```python
from build123d import *

# Parameters (mm, degrees)
F0_R     = 95.25
F0_R_2   = 31.75
F1_DEPTH = 50.8


with BuildPart() as f1:
    # F0 (on Front) → F1 (new body)
    with BuildSketch(Plane.XZ):
        Circle(F0_R)
        with BuildLine():
            ThreePointArc((46.990183, 59.986354), (65.491159, 38.953153), (75.141667, 12.655826))
            ThreePointArc((75.141667, 12.655826), (84.797941, 9.346947), (88.9, 0))
            ThreePointArc((88.9, 0), (84.797941, -9.346947), (75.141667, -12.655826))
            ThreePointArc((75.141667, -12.655826), (65.407135, -39.094076), (46.731427, -60.188153))
            ThreePointArc((46.731427, -60.188153), (48.087021, -63.052889), (48.552253, -66.187838))
            ThreePointArc((48.552253, -66.187838), (40.152635, -76.713719), (28.025311, -70.85917))
            ThreePointArc((28.025311, -70.85917), (0.009492, -76.199999), (-28.007657, -70.86615))
            ThreePointArc((-28.007657, -70.86615), (-43.08737, -75.575185), (-46.716431, -60.199793))
            ThreePointArc((-46.716431, -60.199793), (-65.887351, -38.279198), (-75.435354, -10.767885))
            ThreePointArc((-75.435354, -10.767885), (-86.995, 0), (-75.435354, 10.767885))
            ThreePointArc((-75.435354, 10.767885), (-66.114858, 37.884899), (-47.432359, 59.637332))
            ThreePointArc((-47.432359, 59.637332), (-43.987261, 75.054986), (-28.852362, 70.526458))
            ThreePointArc((-28.852362, 70.526458), (-0.281663, 76.199479), (28.330193, 70.737827))
            ThreePointArc((28.330193, 70.737827), (40.459969, 76.545328), (48.836928, 66.024629))
            ThreePointArc((48.836928, 66.024629), (48.364923, 62.867446), (46.990183, 59.986354))
        make_face(mode=Mode.SUBTRACT)
        with BuildLine():
            ThreePointArc((75.141667, -12.655826), (63.5, 0), (75.141667, 12.655826))
            ThreePointArc((75.141667, 12.655826), (65.491159, 38.953153), (46.990183, 59.986354))
            ThreePointArc((46.990183, 59.986354), (32.652655, 56.67114), (28.330193, 70.737827))
            ThreePointArc((28.330193, 70.737827), (-0.281663, 76.199479), (-28.852362, 70.526458))
            ThreePointArc((-28.852362, 70.526458), (-28.017299, 68.198506), (-27.733988, 65.741593))
            ThreePointArc((-27.733988, 65.741593), (-35.333668, 55.430339), (-47.432359, 59.637332))
            ThreePointArc((-47.432359, 59.637332), (-66.114858, 37.884899), (-75.435354, 10.767885))
            ThreePointArc((-75.435354, 10.767885), (-68.301064, 7.35791), (-65.405, 0))
            ThreePointArc((-65.405, 0), (-68.301064, -7.35791), (-75.435354, -10.767885))
            ThreePointArc((-75.435354, -10.767885), (-65.887351, -38.279198), (-46.716431, -60.199793))
            ThreePointArc((-46.716431, -60.199793), (-34.607099, -55.867083), (-26.945762, -66.197242))
            ThreePointArc((-26.945762, -66.197242), (-27.214583, -68.591314), (-28.007657, -70.86615))
            ThreePointArc((-28.007657, -70.86615), (0.009492, -76.199999), (28.025311, -70.85917))
            ThreePointArc((28.025311, -70.85917), (32.408308, -56.811228), (46.731427, -60.188153))
            ThreePointArc((46.731427, -60.188153), (65.407135, -39.094076), (75.141667, -12.655826))
        make_face()
        Circle(F0_R_2, mode=Mode.SUBTRACT)
    extrude(amount=F1_DEPTH)


solid = f1.part
```
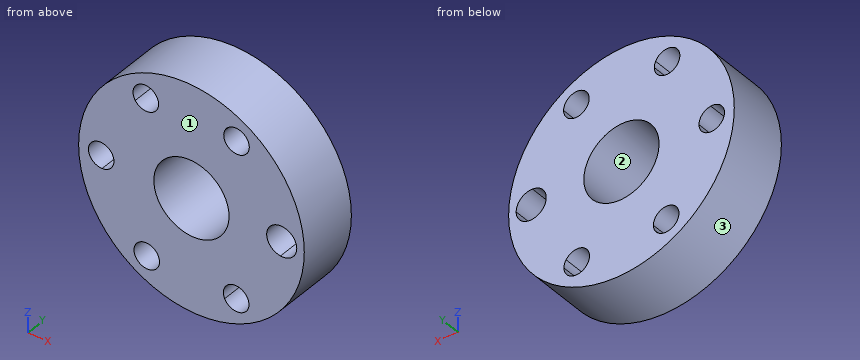
The listing builds one solid part. Answer for the finished solid, in the listing's coordinates (mm). Face numbers are marked on the shaded views. Round coordinates to 2 decimals unless told otherwise and drop trailing zeros. Loops run counter-clockwise (first coordinate to the right, second up) from the corner with the lowest first, then second, coordinate; pieces in that order, holes last. Notation, with made-up numbers: (65, 88.25) - (95, 88.25) arc R13 cw to (95, 105.25) - close; hole circle Ø3 at (-30.5, 55). An arc over 180 degrees is marked (long way). Return JSON: item names as keys, results as strings. Group by question number.
1. The part is cut by section B-B on y = -14.5. Determine the outline of the cut face in (x, z) (3 decimals).
2. The part is cut by section C-C on z = 29.5. Determine the outline of the cut face in (x, y).
3. The part is cut by section D-D on z = 52. Determine the outline of the cut face in (x, y), then the cut area to 3 significant figures.
4. Consider probe 1 along Z at (x, y) = (0, -20); probe 2 along X at (y, z) = (-28, 11); probe 3 along X at (y, z) = (-43, -8.5). Determine where each line is inside the solid, lowest interval first.
5. The mould has two halves that part along X. Classify the marked faces 1, 2 and 3: pulls with the +X half, pulls with the -X half, needs draft (parallel to the pull), parting line crosses it, or undercut.
6. The part is cut by section A-A on x = 0. Determine the outline of the cut face in (y, z), then the cut area to 3 significant figures.
7. Each of these flat-tipped pins is pushed along its axis until it touches: P1, Ø1.5, axis at y = -16, z = -40, coming from the +X side; P2, Ø8, axis at y = -40, z = 63.5, coming from the -X side; P3, Ø8, axis at x = 40.5, y = -32, coming from the +Z side. Where does it stop, or does it pass through?
Resolved:
{
 "1": {"outline": "circle Ø190.5 at (0, 0); hole circle Ø21.59 at (-76.2, 0); hole circle Ø63.5 at (0, 0); hole (-28.852, 70.526) arc R10.795 ccw (long way) to (-27.734, 65.742) arc R10.795 ccw to start; hole (-28.008, -70.866) arc R10.795 ccw to (-26.946, -66.197) arc R10.795 ccw (long way) to start; hole (46.731, -60.188) arc R10.795 ccw (long way) to (48.552, -66.188) arc R10.795 ccw to start; hole (46.99, 59.986) arc R10.795 ccw to (48.837, 66.025) arc R10.795 ccw (long way) to start; hole circle Ø25.4 at (76.2, 0)"},
 "2": {"outline": "(-90.57, -50.8) - (-11.74, -50.8) - (-11.74, 0) - (-90.57, 0) - close; (11.74, -50.8) - (90.57, -50.8) - (90.57, 0) - (11.74, 0) - close"},
 "3": {"outline": "(-79.8, -50.8) - (79.8, -50.8) - (79.8, 0) - (-79.8, 0) - close", "area": "8,110 mm²"},
 "4": {"probe 1": "z = -95.25 to -31.75, 31.75 to 95.25", "probe 2": "x = -94.61 to -29.78, 29.78 to 69.85, 82.55 to 94.61", "probe 3": "x = -94.87 to -82.85, -69.55 to -30.59, 30.59 to 66.76, 85.64 to 94.87"},
 "5": {"face 1": "needs draft", "face 2": "undercut", "face 3": "parting line crosses it"},
 "6": {"outline": "(-50.8, -95.25) - (0, -95.25) - (0, -31.75) - (-50.8, -31.75) - close; (-50.8, 31.75) - (0, 31.75) - (0, 95.25) - (-50.8, 95.25) - close", "area": "6,450 mm²"},
 "7": {"P1": "stops at x = 86.79", "P2": "stops at x = -74.38", "P3": "stops at z = 87.98"}
}
